```python
from build123d import *

# Parameters (mm, degrees)
BOSS_EXTRUDE1_DEPTH = 939.8
SKETCH2_R           = 2.667
BOSS_EXTRUDE2_DEPTH = 3.81
BOSS_EXTRUDE3_START = -3.81
SKETCH3_R           = 2.667
BOSS_EXTRUDE3_DEPTH = 3.81


with BuildPart() as part:
    # Sketch1 → Boss-Extrude1 (new body)
    with BuildSketch(Plane.XY):
        with BuildLine():
            Line((-7.360249805, 3.93392662), (-7.360249805, -3.970205312))
            Line((-7.360249805, -3.970205312), (7.360249805, -3.970205312))
            Line((7.360249805, -3.970205312), (17.707328311, -3.970205312))
            Line((17.707328311, -3.970205312), (14.73419743, -2.484193787))
            Line((14.73419743, -2.484193787), (4.584628721, -2.484193787))
            ThreePointArc((4.584628721, -2.484193787), (-2.195349018, -0.778057865), (-7.360249805, 3.93392662))
        make_face()
    extrude(amount=BOSS_EXTRUDE1_DEPTH)

    # Sketch2 → Boss-Extrude2 (add)
    with BuildSketch(Plane.XY.offset(939.8)):
        with BuildLine():
            Line((-7.360249805, -3.970205312), (0, -3.970205312))
            Line((0, -3.970205312), (0, 7.640068299))
            ThreePointArc((0, 7.640068299), (-0.743948776, 9.436119523), (-2.54, 10.180068299))
            Line((-2.54, 10.180068299), (-7.360249805, 10.180068299))
            Line((-7.360249805, 10.180068299), (-7.360249805, -3.970205312))
        make_face()
        with Locations((-3.81, 6.741214638)):
            Circle(SKETCH2_R, mode=Mode.SUBTRACT)
    extrude(amount=-BOSS_EXTRUDE2_DEPTH)

    # Sketch3 → Boss-Extrude3 (add)
    with BuildSketch(Plane(origin=(0, 0, 0), x_dir=(-1, 0, 0), z_dir=(0, 0, -1)).offset(BOSS_EXTRUDE3_START)):
        with BuildLine():
            Line((0, -1.730708485), (0, -3.970205312))
            Line((0, -3.970205312), (7.360249805, -3.970205312))
            Line((7.360249805, -3.970205312), (7.360249805, 3.93392662))
            Line((7.360249805, 3.93392662), (7.360249805, 10.180068299))
            Line((7.360249805, 10.180068299), (2.54, 10.180068299))
            ThreePointArc((2.54, 10.180068299), (0.743948776, 9.436119523), (0, 7.640068299))
            Line((0, 7.640068299), (0, -1.730708485))
        make_face()
        with Locations(Location((3.81, 6.741214638, 0), (0, 0, 180))):
            Circle(SKETCH3_R, mode=Mode.SUBTRACT)
    extrude(amount=BOSS_EXTRUDE3_DEPTH)


solid = part.part
```
Verification items for the finished model (mm, model axes). Round coordinates to 2 decimals unless told otherwise and drop trailing zeros. Write each loop counter-clockwise with the first axis right and the second up, starting at its lowest first coordinate (ties: lowest second). Pieces come first, ordered by that corner, then holes.
1. Section check A-A on z = 192.5. Enter the section's corners in (x, y), plus the area to 3 significant figures.
2. Gauge pin test, flat ends, axial feed: P1, Ø3, axis at y = 1, z = 937, coming from the +X side; P2, Ø10, axis at x = 15, z = 837, coming from the +Y side; P3, Ø4, axis at x = -2.5, z = 222, coming from the +Y side. Record the tip position at first contact, or that the pin passes through.
3. Section check C-C on x = 8.5. Enter the section's corners in (y, z).
4. Section check B-B on y = 1.25. Enter the section's corners in (x, z).
5. Scan lines: L1, parallel to Y at x = -3.81, z = 937.6; L2, parallel to Y at x = 4.5, z = 58.5; L3, parallel to X at y = -0.5, z = 749. Record each from-to range of solid material in increasing order.
Answer:
1. outline: (-7.36, -3.97) - (17.71, -3.97) - (14.73, -2.48) - (4.58, -2.48) arc R14.32 cw to (-7.36, 3.93) - close
1. area: 57.8 mm2
2. P1: stops at x = 0
2. P2: stops at y = -2.48
2. P3: stops at y = 0.77
3. outline: (-3.97, 0) - (-2.48, 0) - (-2.48, 939.8) - (-3.97, 939.8) - close
4. outline: (-7.36, 0) - (0, 0) - (0, 3.81) - (-5.06, 3.81) - (-5.06, 935.99) - (0, 935.99) - (0, 939.8) - (-7.36, 939.8) - close
5. L1: y = -3.97 to 4.07, 9.41 to 10.18
5. L2: y = -3.97 to -2.48
5. L3: x = -7.36 to -2.69
